from build123d import *

# Parameters (mm, degrees)
SKETCH1_R           = 8.5
SKETCH1_R_2         = 1
SKETCH1_W           = 2.6
SKETCH1_H           = 52
BOSS_EXTRUDE1_DEPTH = 2.5


with BuildPart() as part:
    # Sketch1 → Boss-Extrude1 (new body)
    with BuildSketch(Plane(origin=(0, 0, 0), x_dir=(1, 0, 0), z_dir=(0, 1, 0))):
        Polygon((-25, 35), (-77.6, 35), (-77.6, -35), (-25, -35), (-25, -39), (25, -39), (25, -35), (77.6, -35), (77.6, 35), (25, 35), (25, 39), (-25, 39), align=None)
        with Locations((-12.5, 12.818198975)):
            Circle(SKETCH1_R, mode=Mode.SUBTRACT)
        with Locations((-21, 21.318198975)):
            Circle(SKETCH1_R_2, mode=Mode.SUBTRACT)
        with Locations((-21, 4.318198975)):
            Circle(SKETCH1_R_2, mode=Mode.SUBTRACT)
        with Locations((21, 4.318198975)):
            Circle(SKETCH1_R_2, mode=Mode.SUBTRACT)
        with Locations((21, 21.318198975)):
            Circle(SKETCH1_R_2, mode=Mode.SUBTRACT)
        with Locations((12.5, 12.818198975)):
            Circle(SKETCH1_R, mode=Mode.SUBTRACT)
        with Locations((26, 4.318198975)):
            Circle(SKETCH1_R_2, mode=Mode.SUBTRACT)
        with Locations((34.5, 12.818198975)):
            Circle(SKETCH1_R, mode=Mode.SUBTRACT)
        with Locations((26, 21.318198975)):
            Circle(SKETCH1_R_2, mode=Mode.SUBTRACT)
        with Locations((68, 21.318198975)):
            Circle(SKETCH1_R_2, mode=Mode.SUBTRACT)
        with Locations((68, 4.318198975)):
            Circle(SKETCH1_R_2, mode=Mode.SUBTRACT)
        with Locations((59.5, 12.818198975)):
            Circle(SKETCH1_R, mode=Mode.SUBTRACT)
        with Locations((-68, 4.318198975)):
            Circle(SKETCH1_R_2, mode=Mode.SUBTRACT)
        with Locations((-59.5, 12.818198975)):
            Circle(SKETCH1_R, mode=Mode.SUBTRACT)
        with Locations((-34.5, 12.818198975)):
            Circle(SKETCH1_R, mode=Mode.SUBTRACT)
        with Locations((-26, 21.318198975)):
            Circle(SKETCH1_R_2, mode=Mode.SUBTRACT)
        with Locations((-26, 4.318198975)):
            Circle(SKETCH1_R_2, mode=Mode.SUBTRACT)
        with Locations((-68, 21.318198975)):
            Circle(SKETCH1_R_2, mode=Mode.SUBTRACT)
        with Locations((-73.3, 0)):
            Rectangle(SKETCH1_W, SKETCH1_H, mode=Mode.SUBTRACT)
        with Locations((73.3, 0)):
            Rectangle(SKETCH1_W, SKETCH1_H, mode=Mode.SUBTRACT)
    extrude(amount=BOSS_EXTRUDE1_DEPTH)


solid = part.part
Could you check a few things on this model? Use its own coordinates, in mm. Give positions to 0.01 mm unless a question says otherwise; leave off trailing zeros. Order: outer loops, then holes, each group sorted by start corner. A loop starts at its lowest first (then second) coordinate and runs counter-clockwise, first axis right, second up.
1. Will this pin go through, and if not, where does the flat tip stop? P1, Ø1.2, axis at y = 1, z = -37.5, coming from the -X side.
2. Suppose I cut it at A-A (z = 24.5). List the corners of the cut face in (x, y) for me.
3. We'd pull the mould along X, two halves only. Please class faces 1 (the flat face through (-1, 0, 8)), 2 (the cylindrical face through (-35.607, 1.232, -21.246)): pulls with the +X half, pulls with the -X half, needs draft (parallel to the pull), parting line crosses it, or undercut.
4. Suppose I cut it at C-C (y = 0.55). Give the number of separate pieces and of enclosed holes in the cut face, plus the area to 3 significant figures.
5. Suppose I cut it at B-B (x = 36.5). List the corners of the cut face in (y, z) for me.
6. I need wall thicknesses on L1, parallel to X at y = 1.5, z = 25; L2, parallel to Z at x = 12.5, y = 0.55; L3, parallel to Z at x = 34.5, y = 1.95. Which ranges of each line are inside material? Lowest first, please.
Solved:
1. P1: stops at x = -25
2. outline: (-77.6, 0) - (-74.6, 0) - (-74.6, 2.5) - (-77.6, 2.5) - close; (-72, 0) - (72, 0) - (72, 2.5) - (-72, 2.5) - close; (74.6, 0) - (77.6, 0) - (77.6, 2.5) - (74.6, 2.5) - close
3. face 1: needs draft
3. face 2: undercut
4. separate pieces: 1
4. enclosed holes: 20
4. area: 9,590 mm2
5. outline: (0, -35) - (2.5, -35) - (2.5, -21.08) - (0, -21.08) - close; (0, -4.56) - (2.5, -4.56) - (2.5, 35) - (0, 35) - close
6. L1: x = -77.6 to -74.6, -72 to 72, 74.6 to 77.6
6. L2: z = -39 to -21.32, -4.32 to 39
6. L3: z = -35 to -21.32, -4.32 to 35
